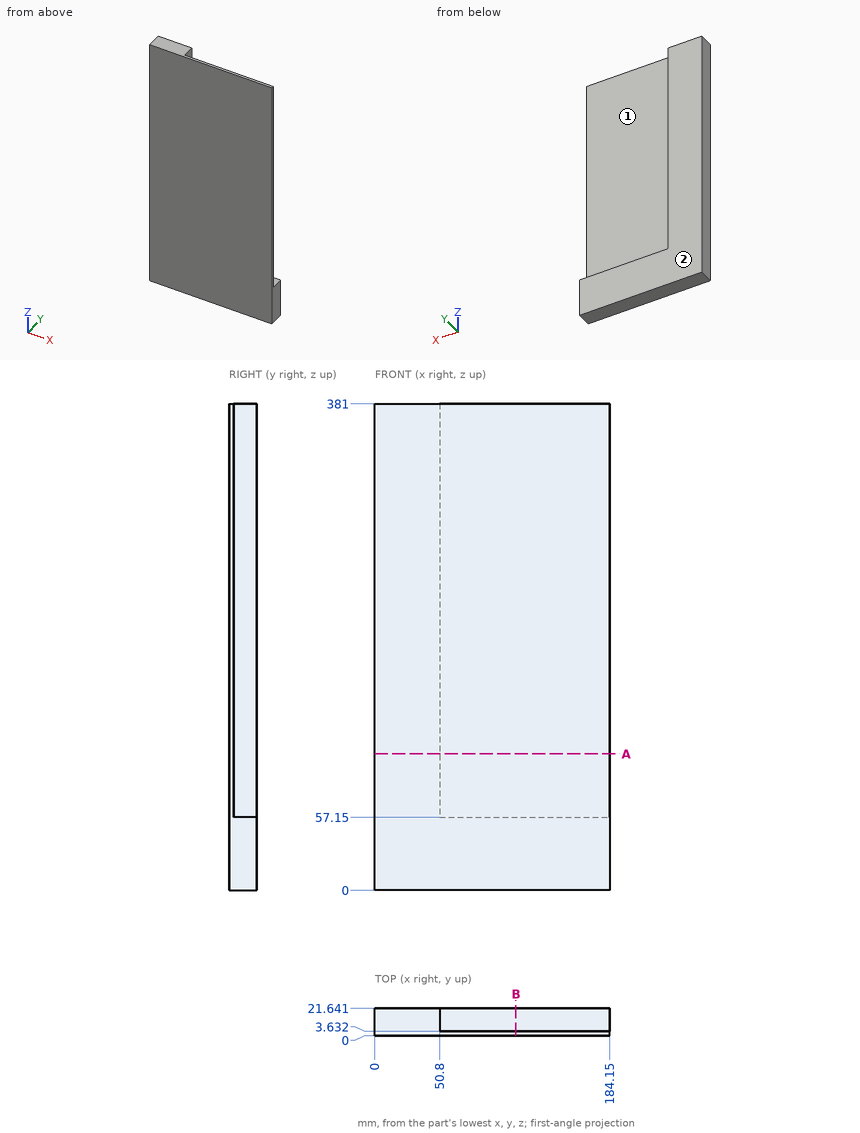
Verification items for this drawing (mm, ordinates from the low corner). A direction names the side the tool comes from. Round coordinates to 2 decimals unless told otherwise and drop trailing zeros. Order: outer loops, then holes, each group sorted by start corner. A loop starts at its lowest first (then second) coordinate and runs counter-clockwise, first axis right, second up. Notation, with made-up numbers: M -22,-30.75 L -12,-30.75 A21 cw -12,8.25 Z; hole C -27.5,15 d5. An arc over 180 degrees is marked long. Answer in a Markdown table with one row per item. Add a question column.
Item 1: Depth check by flat-ended pin: pin 1 Ø4 at (x, y) = (130, 14.5) entering from +Z; pin 2 Ø5.5 at (y, z) = (12.5, 213.5) entering from +X. Enter the tip coordinate at first touch or a pass-through.
Item 2: Material ranges on L1, parallel to X at y = 8, z = 122.5; L2, parallel to Y at x = 152.5, z = 173; L3, parallel to Z at x = 96.5, y = 12, recorded low to high. Write a range as [from, to].
Item 3: Sectioned sample at A-A, the plane z = 107. Enter the section's corners in (x, y).
Item 4: Set-up check for the marked faces 1 and 2: record each of +Z, -Z, +X, -X, +Y, -Y from which the full face is reachable in a straight line by a thin tool's end or side.
Item 5: Sectioned sample at B-B, the plane x = 110.5. Enter the section's corners in (y, z).
Filled in:
| question | item | result |
|---|---|---|
| 1 | pin 1 | stops at z = 57.15 |
| 1 | pin 2 | stops at x = 50.8 |
| 2 | L1 | x = [0, 50.8] |
| 2 | L2 | y = [0, 3.63] |
| 2 | L3 | z = [0, 57.15] |
| 3 | outline | M 0,0 L 184.15,0 L 184.15,3.63 L 50.8,3.63 L 50.8,21.64 L 0,21.64 Z |
| 4 | face 1 | +Z, +X, +Y |
| 4 | face 2 | +Z, -Z, +X, -X, +Y |
| 5 | outline | M 0,0 L 21.64,0 L 21.64,57.15 L 3.63,57.15 L 3.63,381 L 0,381 Z |
